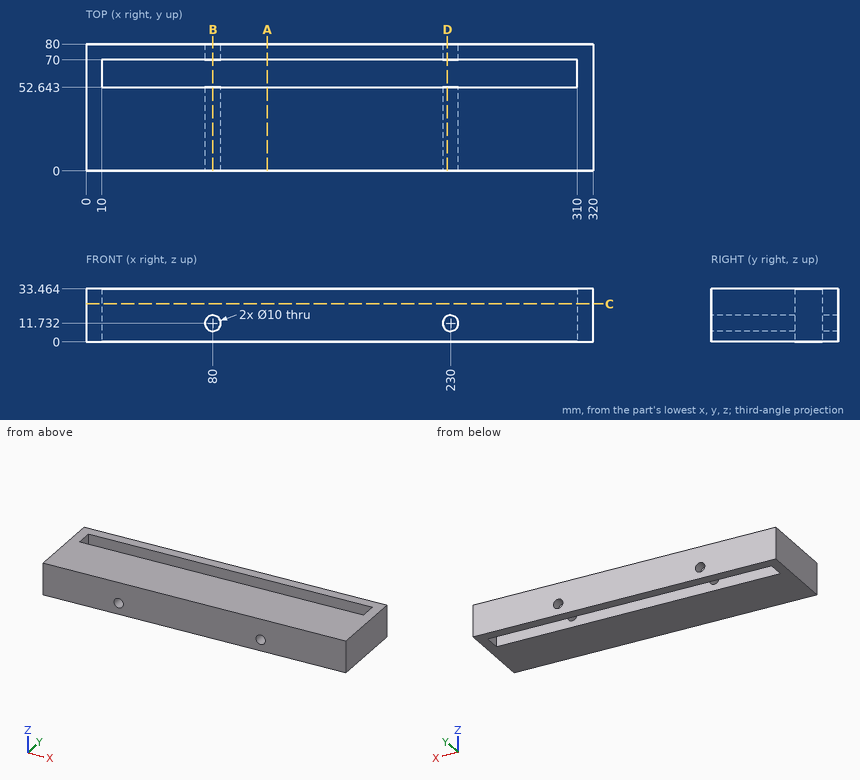
Could you check a few things on this drawing? It's one solid part, dimensions in mm from its lowest x, y, z. Give positions to 0.01 mm unless a question says otherwise; leave off trailing zeros. Order: outer loops, then holes, each group sorted by start corner. A loop starts at its lowest first (then second) coordinate and runs counter-clockwise, first axis right, second up. Notation, with made-up numbers: (53.25, -38.75) - (71.25, -38.75) arc R22 ccw to (71.25, -2.75) - close; hole circle Ø8 at (-26.5, -10). An arc over 180 degrees is marked (long way). Answer as a JSON object with one key per item and string values. Group by question number.
Item 1: If we section it at A-A on x = 114.5: Please give me the cut outline in (y, z) (1 decimal), and give its area (3 significant figures).
Item 2: Please list where these lines run through material, in increasing order: probe 1 along Y at (x, z) = (14.5, 6); probe 2 along X at (y, z) = (53, 26.5); probe 3 along Z at (x, y) = (80, 27) (1 decimal).
Item 3: If we section it at B-B on x = 80: Please give me the cut outline in (y, z) (1 decimal).
Item 4: If we section it at D-D on x = 228: Give the number of separate pieces and of enclosed holes in the cut face, and give its area (3 significant figures).
Item 5: If we section it at C-C on z = 24: Please give me the cut outline in (x, y), and give its area (3 significant figures).
Result set:
{
 "1": {"outline": "(0, 0) - (52.6, 0) - (52.6, 33.5) - (0, 33.5) - close; (70, 0) - (80, 0) - (80, 33.5) - (70, 33.5) - close", "area": "2,100 mm²"},
 "2": {"probe 1": "0 to 52.64, 70 to 80", "probe 2": "0 to 10, 310 to 320", "probe 3": "0 to 6.7, 16.7 to 33.5"},
 "3": {"outline": "(0, 0) - (52.6, 0) - (52.6, 6.7) - (0, 6.7) - close; (0, 16.7) - (52.6, 16.7) - (52.6, 33.5) - (0, 33.5) - close; (70, 0) - (80, 0) - (80, 6.7) - (70, 6.7) - close; (70, 16.7) - (80, 16.7) - (80, 33.5) - (70, 33.5) - close"},
 "4": {"separate pieces": "4", "enclosed holes": "0", "area": "1,520 mm²"},
 "5": {"outline": "(0, 0) - (320, 0) - (320, 80) - (0, 80) - close; hole (10, 52.64) - (310, 52.64) - (310, 70) - (10, 70) - close", "area": "20,400 mm²"}
}
